Answer from the drawing. Dimensions are ordinates in mm from the lowest x, y and z of the part. A direction names the side the tool comes from. Give positions to 0.01 mm unless a question says otherwise; leave off trailing zeros. Write each loop counter-clockwise with the first axis right and the second up, starting at its lowest first coordinate (ties: lowest second). Pieces come first, ordered by that corner, then holes. Notation, with made-up numbers: (72, -23.5) -> (98, -23.5) arc R19 cw to (98, -13.5) -> close; hole circle Ø1 at (42.25, 54). An arc over 180 degrees is marked (long way). Use a Markdown table: item, result. Add a question column.
Q1. For a pull along Y with two mould halves and no side action, classify the marked faces 1, 2 and 3 as pulls with the +Y half, pulls with the -Y half, needs draft (parallel to the pull), parting line crosses it, or undercut.
Q2. For the marked faces 4 and 5, determine the directions among +Z, -Z, +X, -X, +Y, -Y from which every point of the face is accessible in a straight line to the end or side of a thin tool.
Q3. Consider line 1 (Z direction, x = 3.3, y = 0.3); line 2 (Y direction, x = 2.9, z = 1.4); line 3 (Y direction, x = 2.9, z = 3.7). Determine where each line is inside the solid, lowest interval first.
Q4. Section D-D, the plane y = 1.2 is taken. Give the vertices of the cut face in (x, z), plus the area to 3 significant figures.
Q5. Section A-A, the plane x = 2.9 is taken. Give the vertices of the cut face in (y, z), plus the area to 3 significant figures.
Q6. Each of these flat-tipped pins is pushed along its axis until it touches: pin 1 Ø1.5 at (y, z) = (5, 2.5) entering from +X; pin 2 Ø1 at (x, z) = (4, 1) entering from -Y; pin 3 Ø1.5 at (x, z) = (3, 2.5) entering from -Y. Where does it stop, or does it pass through?
Q7. Section C-C, the plane z = 2.6 is taken. Give the vertices of the cut face in (x, y), plus the area to 3 significant figures.
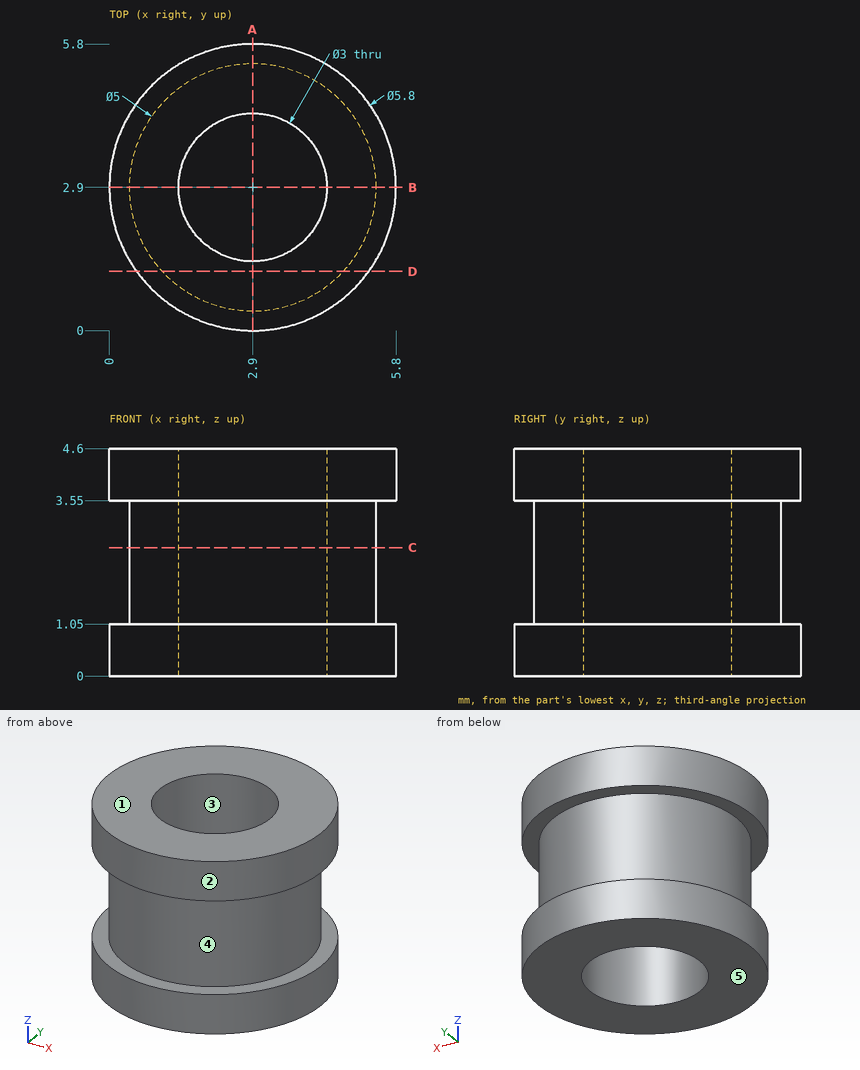
Result set:
| question | item | result |
|---|---|---|
| 1 | face 1 | needs draft |
| 1 | face 2 | parting line crosses it |
| 1 | face 3 | undercut |
| 2 | face 4 | none |
| 2 | face 5 | -Z, +X, -X, +Y, -Y |
| 3 | line 1 | z = 0 to 1.05, 3.55 to 4.6 |
| 3 | line 2 | y = 0.4 to 1.4, 4.4 to 5.4 |
| 3 | line 3 | y = 0 to 1.4, 4.4 to 5.8 |
| 4 | outline | (0.55, 0) -> (5.25, 0) -> (5.25, 1.05) -> (4.73, 1.05) -> (4.73, 3.55) -> (5.25, 3.55) -> (5.25, 4.6) -> (0.55, 4.6) -> (0.55, 3.55) -> (1.07, 3.55) -> (1.07, 1.05) -> (0.55, 1.05) -> close |
| 4 | area | 19.0 mm2 |
| 5 | outline | (0, 0) -> (1.4, 0) -> (1.4, 4.6) -> (0, 4.6) -> (0, 3.55) -> (0.4, 3.55) -> (0.4, 1.05) -> (0, 1.05) -> close; (4.4, 0) -> (5.8, 0) -> (5.8, 1.05) -> (5.4, 1.05) -> (5.4, 3.55) -> (5.8, 3.55) -> (5.8, 4.6) -> (4.4, 4.6) -> close |
| 5 | area | 10.9 mm2 |
| 6 | pin 1 | stops at x = 5 |
| 6 | pin 2 | stops at y = 0.06 |
| 6 | pin 3 | stops at y = 0.4 |
| 7 | outline | circle Ø5 at (2.9, 2.9); hole circle Ø3 at (2.9, 2.9) |
| 7 | area | 12.6 mm2 |
